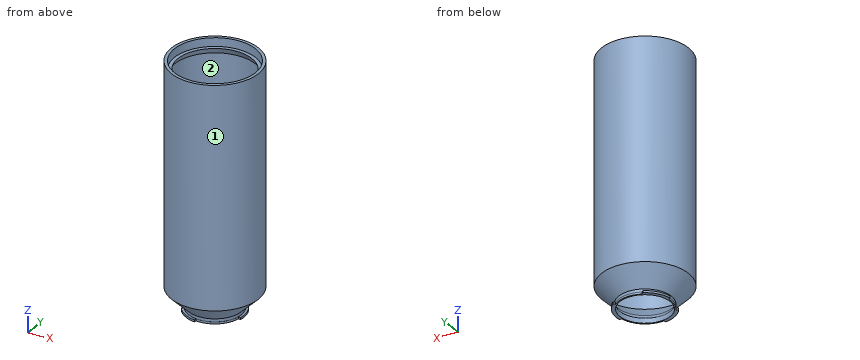
```python
from build123d import *

# Parameters (mm, degrees)
F0_R     = 20.8
F1_DEPTH = 1.65
F2_R     = 21.79
F2_R_2   = 20.8
F3_DEPTH = 2.42


with BuildPart() as f1:
    # F0 (on Top) → F1 (new body)
    with BuildSketch(Plane.XY):
        with BuildLine():
            Line((-23.346566, 4.62362), (-21.59853, 3.30545))
            ThreePointArc((-21.59853, 3.30545), (-21.304567, -4.85159), (-18.037579, -12.331596))
            Line((-18.037579, -12.331596), (-19.64734, -13.432127))
            ThreePointArc((-19.64734, -13.432127), (-12.319875, -20.363219), (-2.779779, -23.637107))
            Line((-2.779779, -23.637107), (-2.779779, -21.672456))
            ThreePointArc((-2.779779, -21.672456), (12.912471, -17.626417), (21.501922, -3.884566))
            Line((21.501922, -3.884566), (23.420858, -4.231244))
            ThreePointArc((23.420858, -4.231244), (22.459544, 7.874571), (15.650801, 17.93021))
            Line((15.650801, 17.93021), (14.368487, 16.461138))
            ThreePointArc((14.368487, 16.461138), (3.12676, 21.625121), (-9.117285, 19.856928))
            Line((-9.117285, 19.856928), (-10.865321, 21.175098))
            ThreePointArc((-10.865321, 21.175098), (-19.002662, 14.329649), (-23.346566, 4.62362))
        make_face()
        Circle(F0_R, mode=Mode.SUBTRACT)
    extrude(amount=F1_DEPTH)

    # F2 (on face) → F3 (join)
    with BuildSketch(Plane.XY.offset(1.65)):
        Circle(F2_R)
        Circle(F2_R_2, mode=Mode.SUBTRACT)
    extrude(amount=F3_DEPTH)

    # F4 (on Right) → F5 (revolve)
    with BuildSketch(Plane.YZ):
        Polygon((-33.5, 193), (-33.5, 200), (-36, 200), (-36, 18.28), (-21.79, 4.07), (-20.8, 4.07), (-22.147417, 6.927417), (-33.5, 18.28), (-33.5, 187.803848), (-30.5, 193), align=None)
    revolve(axis=Axis((0, 0, 100), (0, 0, 1)))


solid = f1.part
```
Check sheet for the modelled part. Datum: model origin and axes. Units: mm. Face numbers are marked on the shaded views. Coordinates: 2 decimals unless noted, no trailing zeros. Order: outer loops, then holes, each group sorted by start corner. A loop starts at its lowest first (then second) coordinate and runs counter-clockwise, first axis right, second up. Notation, with made-up numbers: M -13,-14 L 43,-14 A12 ccw 43,-6 Z; hole C 0,-35 d4. An arc over 180 degrees is marked long. One line per question, with ' | ' between items. Start each with the question number.
Item 1: Sectioned sample at A-A on y = 0. Record the cut outline in (x, z), and give its area (3 significant figures).
Item 2: Material ranges on line 1 (X direction, y = 0, z = 70); line 2 (Y direction, x = 0, z = 3.05), recorded low to high.
Item 3: Mould release check, pull along X, two halves, no side actions. Record for the marked faces 1 and 2: pulls with the +X half, pulls with the -X half, needs draft (parallel to the pull), parting line crosses it, or undercut.
Item 4: Sectioned sample at B-B on x = 0. Record the cut outline in (y, z).
Item 5: Gauge pin test, flat ends, axial feed: P1, Ø6, axis at x = 4, y = 28, coming from the +Z side; P2, Ø6, axis at y = 16, z = 24, coming from the -X side; P3, Ø1, axis at x = -9.5, y = -25.5, coming from the -Z side; P4, Ø22.5, axis at x = 6.5, y = 1, coming from the +Z side. Record the tip position at first contact, or that the pin passes through.
Item 6: Sectioned sample at C-C on z = 151.5. Record the cut outline in (x, y).
Answer below:
1) outline: M -36,18.28 L -21.79,4.07 L -21.79,1.65 L -21.85,1.65 L -21.85,0 L -20.8,0 L -20.8,4.07 L -22.15,6.93 L -33.5,18.28 L -33.5,187.8 L -30.5,193 L -33.5,193 L -33.5,200 L -36,200 Z; M 20.8,0 L 23.8,0 L 23.8,1.65 L 21.79,1.65 L 21.79,4.07 L 36,18.28 L 36,200 L 33.5,200 L 33.5,193 L 30.5,193 L 33.5,187.8 L 33.5,18.28 L 22.15,6.93 L 20.8,4.07 Z | area: 1,000 mm^2
2) line 1: x = -36 to -33.5, 33.5 to 36 | line 2: y = -21.79 to -20.8, 20.8 to 21.79
3) face 1: parting line crosses it | face 2: undercut
4) outline: M -36,18.28 L -21.79,4.07 L -21.79,1.65 L -21.85,1.65 L -21.85,0 L -20.8,0 L -20.8,4.07 L -22.15,6.93 L -33.5,18.28 L -33.5,187.8 L -30.5,193 L -33.5,193 L -33.5,200 L -36,200 Z; M 20.8,0 L 21.85,0 L 21.85,1.65 L 21.79,1.65 L 21.79,4.07 L 36,18.28 L 36,200 L 33.5,200 L 33.5,193 L 30.5,193 L 33.5,187.8 L 33.5,18.28 L 22.15,6.93 L 20.8,4.07 Z
5) P1: stops at z = 193 | P2: stops at x = -33.57 | P3: stops at z = 8.99 | P4: passes through
6) outline: C 0,0 d72; hole C 0,0 d67
